Geometry: see drawing. Coordinates: mm, zero at the bounding-box minimum. Coordinates: 2 decimals unless noted, no trailing zeros. Write each loop counter-clockwise with the first axis right and the second up, starting at its lowest first coordinate (ties: lowest second). Pieces come first, ordered by that corner, then holes. Notation, with made-up numbers: (-15.5, 43) -> (30.5, 43) arc R26 ccw to (30.5, 78) -> close; hole circle Ø1 at (4, 77). An arc over 180 degrees is marked (long way). Use one line per item in the form item = value. Start each with the question number.
(1) Cut plane C-C on z = 4.5. Return the cut outline in (x, y), plus the area to 3 significant figures.
(2) Cut plane A-A on x = 15. Return the cut outline in (y, z).
(3) Ray query, line 1 along Y through (x, z) = (15, 2.75); line 2 along Y through (x, z) = (13.5, 0.5); line 3 along X through (y, z) = (13.5, 3.25). Return the intervals inside material, ascending.
(4) Cut plane B-B on y = 125. Return the cut outline in (x, z), plus the area to 3 significant figures.
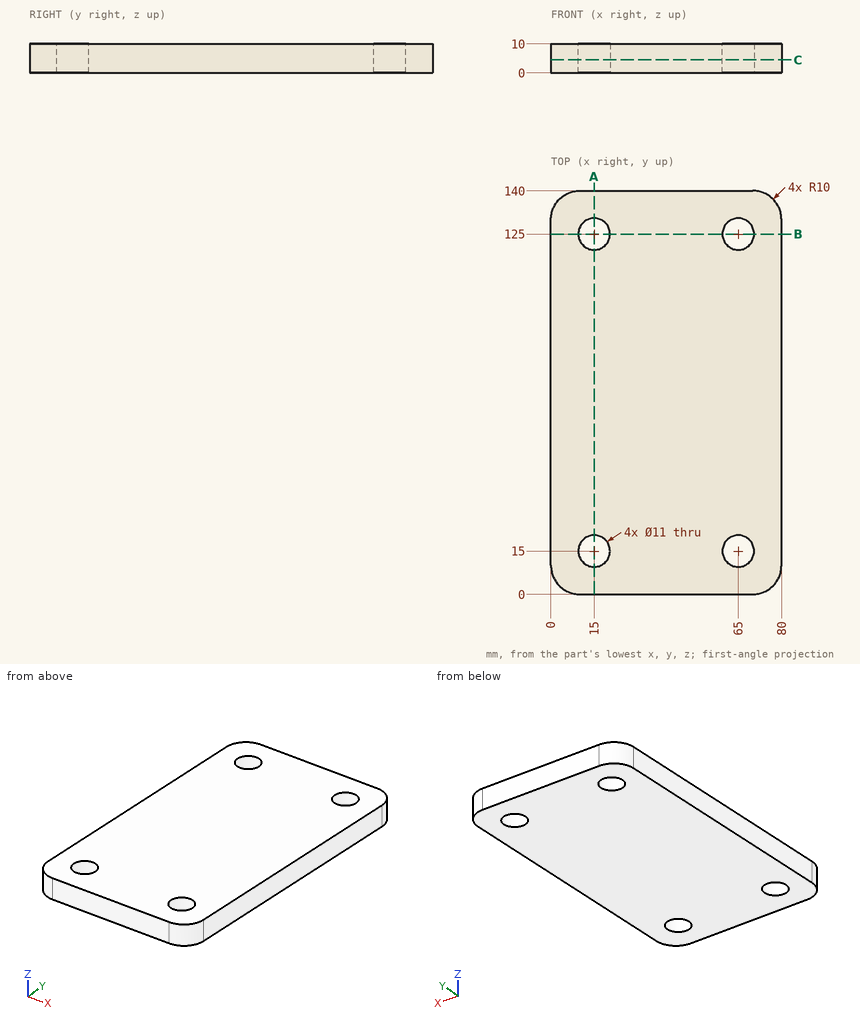
Values:
q1.outline = (0, 10) arc R10 ccw to (10, 0) -> (70, 0) arc R10 ccw to (80, 10) -> (80, 130) arc R10 ccw to (70, 140) -> (10, 140) arc R10 ccw to (0, 130) -> close; hole circle Ø11 at (15, 15); hole circle Ø11 at (15, 125); hole circle Ø11 at (65, 15); hole circle Ø11 at (65, 125)
q1.area = 10,700 mm2
q2.outline = (0, 0) -> (9.5, 0) -> (9.5, 10) -> (0, 10) -> close; (20.5, 0) -> (119.5, 0) -> (119.5, 10) -> (20.5, 10) -> close; (130.5, 0) -> (140, 0) -> (140, 10) -> (130.5, 10) -> close
q3.line_1 = 0 to 9.5, 20.5 to 119.5, 130.5 to 140
q3.line_2 = 0 to 9.71, 20.29 to 119.71, 130.29 to 140
q3.line_3 = 0 to 9.71, 20.29 to 59.71, 70.29 to 80
q4.outline = (0, 0) -> (9.5, 0) -> (9.5, 10) -> (0, 10) -> close; (20.5, 0) -> (59.5, 0) -> (59.5, 10) -> (20.5, 10) -> close; (70.5, 0) -> (80, 0) -> (80, 10) -> (70.5, 10) -> close
q4.area = 580 mm2
